Input: part model. Units: mm. Frame: model coordinates. Face numbers are marked on the shaded views. Round coordinates to 2 decimals unless told otherwise and drop trailing zeros. Write each loop counter-clockwise with the first axis right and the second up, starting at its lowest first coordinate (ties: lowest second). Pieces come first, ordered by that corner, then holes. Notation, with made-up numbers: (45, 10) - (63, 10) arc R12 cw to (63, 26) - close; hole circle Ø11 at (28, 83.25). An arc over 180 degrees is marked (long way). One line per item, written item: value. Start each with the question number.
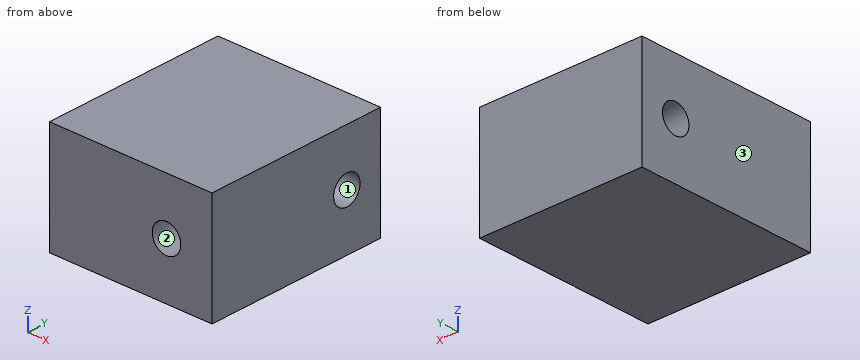
Autodesk Inventor part; units mm, degrees
ref_plane "YZ Plane" through (0, 0, 0) normal (1, 0, 0) x (0, 1, 0)
ref_plane "XZ Plane" through (0, 0, 0) normal (0, 1, 0) x (-1, 0, 0)
ref_plane "XY Plane" through (0, 0, 0) normal (0, 0, 1) x (1, 0, 0)
sketch "Sketch1" plane through (0, 0, 0) normal (1, 0, 0) x (0, 1, 0)
  line L0 (0, 0) -> (31.75, 0)
  line L1 (31.75, 0) -> (31.75, -19.05)
  line L2 (31.75, -19.05) -> (0, -19.05)
  line L3 (0, -19.05) -> (0, 0)
  circle A0 centre (25.4, -9.525) radius 3.2512 construction
  dimension "d0" = 31.75
  dimension "d1" = 19.05
  dimension "d2" = 6.5024
  dimension "d3" = 6.35
  dimension "d4" = 9.525
extrude "Extrusion1" add sketch "Sketch1" along normal blind 28.4226
hole "Hole1" at (0, 25.4, -9.525) at (0, 25.4, -9.525) direction (1, 0, 0) diameter 4.9784 end through all
sketch "Sketch2" plane through (0, 0, -19.05) normal (0, -1, 0) x (1, 0, 0)
  line L0 (0, 19.05) -> (0, 0)
  line L1 (0, 0) -> (28.4226, 0)
  line L2 (28.4226, 19.05) -> (28.4226, 0)
  line L3 (0, 19.05) -> (28.4226, 19.05)
  line L4 (28.4226, 2.307) -> (7.7724, 2.307) construction
  point P0 (20.4724, 9.525)
  dimension "d14" = 20.6502
  dimension "d15" = 7.9502
  dimension "d16" = 9.525
hole "Hole2" at (20.4724, 0, -9.525) direction (0, 1, 0) diameter 4.9784 depth 19.05
properties part number "Intake Pivot Billet" material "Aluminum 6061"
Q1. Pull-direction query (X, two-part tool) for the marked faces 1, 2 and 3; classes: pulls with the +X half, pulls with the -X half, needs draft (parallel to the pull), parting line crosses it, or undercut.
Q2. Cut plane A-A, the plane y = 25.4. Output: boundary loops of the cut face in (x, z).
Q3. Cut plane C-C, the plane z = -10.75. Output: boundary loops of the cut face in (x, y), and give its area (3 significant figures).
Q4. Cut plane D-D, the plane y = 6. Output: boundary loops of the cut face in (x, z) (3 decimals), and give its area (3 significant figures).
Q5. Material intervals for probe 1 along Z at (x, y) = (10.75, 25.4); probe 2 along Y at (x, z) = (11.5, -9.5); probe 3 along Y at (x, z) = (15, -10.25), sorted ascending. Write a range as from..to.
Q6. Cut plane B-B, the plane x = 15.25. Output: boundary loops of the cut face in (y, z) (3 decimals), and give its area (3 significant figures).
A:
1. face 1: needs draft
1. face 2: undercut
1. face 3: pulls with the -X half
2. outline: (0, -19.05) - (28.42, -19.05) - (28.42, -12.01) - (0, -12.01) - close; (0, -7.04) - (28.42, -7.04) - (28.42, 0) - (0, 0) - close
3. outline: (0, 0) - (18.31, 0) - (18.31, 19.05) - (22.64, 19.05) - (22.64, 0) - (28.42, 0) - (28.42, 23.23) - (0, 23.23) - close; (0, 27.57) - (28.42, 27.57) - (28.42, 31.75) - (0, 31.75) - close
3. area: 697 mm²
4. outline: (0, -19.05) - (28.423, -19.05) - (28.423, 0) - (0, 0) - close; hole circle Ø4.978 at (20.472, -9.525)
4. area: 522 mm²
5. probe 1: z = -19.05..-12.01, -7.04..0
5. probe 2: y = 0..22.91, 27.89..31.75
5. probe 3: y = 0..23.02, 27.78..31.75
6. outline: (0, -19.05) - (31.75, -19.05) - (31.75, 0) - (0, 0) - close; hole circle Ø4.978 at (25.4, -9.525)
6. area: 585 mm²
